from build123d import *

# Parameters (mm, degrees)
BOSS_EXTRUDE1_DEPTH = 50
SKETCH3_R           = 2.5
CUT_EXTRUDE1_DEPTH  = 24


with BuildPart() as part:
    # Sketch1 → Boss-Extrude1 (new body)
    with BuildSketch(Plane.XY):
        with BuildLine():
            Line((-20, -165), (0, -165))
            Line((0, -165), (0, -172.5))
            Line((0, -172.5), (-51.3765108, -172.5))
            Line((-51.3765108, -172.5), (-65, -172.5))
            ThreePointArc((-65, -172.5), (-86.213203436, -163.713203436), (-95, -142.5))
            Line((-95, -142.5), (-95, -22.5))
            ThreePointArc((-95, -22.5), (-86.213203436, -1.286796564), (-65, 7.5))
            Line((-65, 7.5), (-55, 7.5))
            Line((-55, 7.5), (0, 7.5))
            Line((0, 7.5), (0, 0))
            Line((0, 0), (-55, 0))
            ThreePointArc((-55, 0), (-76.213203436, -8.786796564), (-85, -30))
            Line((-85, -30), (-85, -135))
            ThreePointArc((-85, -135), (-76.213203436, -156.213203436), (-55, -165))
            Line((-55, -165), (-20, -165))
        make_face()
    extrude(amount=BOSS_EXTRUDE1_DEPTH)

    # Sketch3 → Cut-Extrude1 (cut)
    with BuildSketch(Plane.XZ):
        with Locations(Location((-20, 35, 0), (0, 0, 270))):
            Circle(SKETCH3_R)
        with Locations(Location((-20, 15, 0), (0, 0, 270))):
            Circle(SKETCH3_R)
    extrude(amount=-CUT_EXTRUDE1_DEPTH, mode=Mode.SUBTRACT)


solid = part.part
Here's how the part is built. I have some questions about the finished solid (model axes, mm). A direction names the side the tool comes from. Give positions to 0.01 mm unless a question says otherwise; leave off trailing zeros. Loops run counter-clockwise (first coordinate to the right, second up) from the corner with the lowest first, then second, coordinate; pieces in that order, holes last. Notation, with made-up numbers: (39.5, 0) -> (88.5, 0) arc R15 cw to (88.5, 18) -> close; hole circle Ø1 at (34, 66). An arc over 180 degrees is marked (long way). One line per item, written item: value.
Q1. I'm going to push a flat-ended pin straight in: pin 1 Ø2 at (y, z) = (-133, 35.5) entering from +X. Where does the tip first touch, or does it pass through?
Answers follow:
pin 1: x = -85
Q2. Suppose I cut it at B-B on z = 35. Please give me the cut outline in (x, y), then the cut area to 3 significant figures.
Answers follow:
outline: (-95, -142.5) arc R30 ccw to (-65, -172.5) -> (0, -172.5) -> (0, -165) -> (-55, -165) arc R30 cw to (-85, -135) -> (-85, -30) arc R30 cw to (-55, 0) -> (-22.5, 0) -> (-22.5, 7.5) -> (-65, 7.5) arc R30 ccw to (-95, -22.5) -> close; (-17.5, 0) -> (0, 0) -> (0, 7.5) -> (-17.5, 7.5) -> close
area: 3,040 mm^2
Q3. If I drill on line 1 along Y through (x, z) = (-22, 6); line 2 along X through (y, z) = (-118.5, 30.5); line 3 along Y through (x, z) = (-75, 4), over which ranges is the centre line in solid material (lowest first)?
Answers follow:
line 1: -172.5 to -165, 0 to 7.5
line 2: -95 to -85
line 3: -170.78 to -157.36, -7.64 to 5.78
Q4. We'd pull the mould along Z, two halves only. Please class faces 3 (the face through (-86, -89, 0)), 4 (the face through (-19.249, 3.697, 32.615)), 5 (the face through (0, 4, 25)), 6 (the face through (-18.31, 3.7, 16.84)): pulls with the +Z half, pulls with the -Z half, needs draft (parallel to the pull), parting line crosses it, or undercut.
Answers follow:
face 3: pulls with the -Z half
face 4: undercut
face 5: needs draft
face 6: undercut
Q5. Suppose I cut it at C-C on z = 19.5. Please give me the cut outline in (x, y).
Answers follow:
outline: (-95, -142.5) arc R30 ccw to (-65, -172.5) -> (0, -172.5) -> (0, -165) -> (-55, -165) arc R30 cw to (-85, -135) -> (-85, -30) arc R30 cw to (-55, 0) -> (0, 0) -> (0, 7.5) -> (-65, 7.5) arc R30 ccw to (-95, -22.5) -> close
Q6. On a 3-axis mill with a long thin cutter (end or side, diameter ignored), from which of +Z, -Z, +X, -X, +Y, -Y can I reach the whole of each face in a straight line? I mean faces 1 (the face through (-28, -165, 25)), 2 (the face through (-95, -83, 25)). Say none if no direction works.
Answers follow:
face 1: +Z, -Z, +X
face 2: +Z, -Z, -X, +Y, -Y
Q7. Suppose I cut it at D-D on y = -80. Please give me the cut outline in (x, z).
Answers follow:
outline: (-95, 0) -> (-85, 0) -> (-85, 50) -> (-95, 50) -> close
Q8. Suppose I cut it at A-A on x = -27. Please give me the cut outline in (y, z).
Answers follow:
outline: (-172.5, 0) -> (-165, 0) -> (-165, 50) -> (-172.5, 50) -> close; (0, 0) -> (7.5, 0) -> (7.5, 50) -> (0, 50) -> close
